Check sheet for the modelled part. Datum: model origin and axes. Units: mm. Face numbers are marked on the shaded views. A direction names the side the tool comes from. Round coordinates to 2 decimals unless told otherwise and drop trailing zeros. Write each loop counter-clockwise with the first axis right and the second up, starting at its lowest first coordinate (ties: lowest second). Pieces come first, ordered by that corner, then holes. Notation, with made-up numbers: M 12,17 L 22,17 A26 cw 22,37 Z; hole C 40,-19.5 d1. An arc over 180 degrees is marked long. One line per item, written item: value.
from build123d import *

# Parameters (mm, degrees)
SKETCH1_W           = 10.795
SKETCH1_H           = 10.795
BOSS_EXTRUDE1_DEPTH = 6.2992
SKETCH3_R           = 5.7404
BOSS_EXTRUDE2_DEPTH = 3
SKETCH4_R           = 2.8194
BOSS_EXTRUDE3_DEPTH = 19.939
SKETCH5_R           = 0.8255
CUT_EXTRUDE1_DEPTH  = 15
SKETCH7_R           = 3.2385
BOSS_EXTRUDE4_DEPTH = 10
SKETCH8_W           = 4.31
SKETCH8_H           = 1.016
BOSS_EXTRUDE5_DEPTH = 1


with BuildPart() as part:
    # Sketch1 → Boss-Extrude1 (new body)
    with BuildSketch(Plane(origin=(0, 0, 0), x_dir=(1, 0, 0), z_dir=(0, 1, 0))):
        Rectangle(SKETCH1_W, SKETCH1_H)
    extrude(amount=BOSS_EXTRUDE1_DEPTH)

    # Sketch3 → Boss-Extrude2 (add)
    with BuildSketch(Plane(origin=(0, 6.2992, 0), x_dir=(1, 0, 0), z_dir=(0, 1, 0))):
        Circle(SKETCH3_R)
    extrude(amount=-BOSS_EXTRUDE2_DEPTH)

    # Sketch4 → Boss-Extrude3 (add)
    with BuildSketch(Plane(origin=(0, 0, 0), x_dir=(1, 0, 0), z_dir=(0, 1, 0))):
        Circle(SKETCH4_R)
    extrude(amount=BOSS_EXTRUDE3_DEPTH)

    # Sketch5 → Cut-Extrude1 (cut)
    with BuildSketch(Plane(origin=(0, 19.939, 0), x_dir=(1, 0, 0), z_dir=(0, 1, 0))):
        Circle(SKETCH5_R)
    extrude(amount=-CUT_EXTRUDE1_DEPTH, mode=Mode.SUBTRACT)

    # Sketch7 → Boss-Extrude4 (add)
    with BuildSketch(Plane(origin=(0, 0, 0), x_dir=(1, 0, 0), z_dir=(0, 1, 0))):
        Circle(SKETCH7_R)
    extrude(amount=BOSS_EXTRUDE4_DEPTH)

    # Sketch8 → Boss-Extrude5 (add)
    with BuildSketch(Plane(origin=(0, 0, 0), x_dir=(1, 0, 0), z_dir=(0, 1, 0))):
        with Locations((-7.0525, 3.81)):
            Rectangle(SKETCH8_W, SKETCH8_H)
        with Locations((-7.0525, 1.27)):
            Rectangle(SKETCH8_W, SKETCH8_H)
        with Locations((-7.0525, -1.27)):
            Rectangle(SKETCH8_W, SKETCH8_H)
        with Locations((-7.0525, -3.81)):
            Rectangle(SKETCH8_W, SKETCH8_H)
        with Locations((7.0525, -3.81)):
            Rectangle(SKETCH8_W, SKETCH8_H)
        with Locations((7.0525, -1.27)):
            Rectangle(SKETCH8_W, SKETCH8_H)
        with Locations((7.0525, 1.27)):
            Rectangle(SKETCH8_W, SKETCH8_H)
        with Locations((7.0525, 3.81)):
            Rectangle(SKETCH8_W, SKETCH8_H)
    extrude(amount=BOSS_EXTRUDE5_DEPTH)


solid = part.part
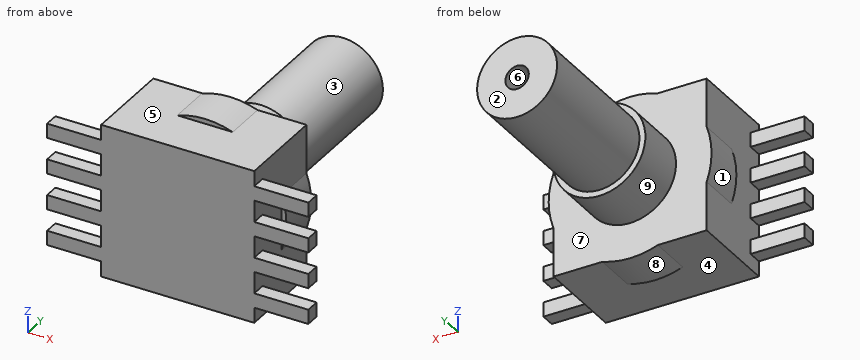
Q1. Scan lines: line 1 (X direction, y = 14.75, z = 0); line 2 (Y direction, x = -0.75, z = 4.5). Record each from-to range of solid material in increasing order. Write a range as [from, to].
Completed:
line 1: [-2.82, -0.83], [0.83, 2.82]
line 2: [0, 6.3]
Q2. Sectioned sample at C-C on y = 5.25. Enter the section's corners in (x, z).
Completed:
outline: M -5.4,-5.4 L -1.95,-5.4 A5.74 ccw 1.95,-5.4 L 5.4,-5.4 L 5.4,-1.95 A5.74 ccw 5.4,1.95 L 5.4,5.4 L 1.95,5.4 A5.74 ccw -1.95,5.4 L -5.4,5.4 L -5.4,1.95 A5.74 ccw -5.4,-1.95 Z
Q3. Draft check along Z on the marked faces 6, 7, 8 and 9. Enter one of: pulls with the +Z half, pulls with the -Z half, needs draft (parallel to the pull), parting line crosses it, or undercut.
Completed:
face 6: undercut
face 7: needs draft
face 8: pulls with the -Z half
face 9: parting line crosses it
Q4. Sectioned sample at D-D on x = 0. Enter the section's corners in (y, z), and give its area (3 significant figures).
Completed:
outline: M 0,-5.4 L 3.3,-5.4 L 3.3,-5.74 L 6.3,-5.74 L 6.3,-3.24 L 10,-3.24 L 10,-2.82 L 19.94,-2.82 L 19.94,-0.83 L 10,-0.83 L 10,0.83 L 19.94,0.83 L 19.94,2.82 L 10,2.82 L 10,3.24 L 6.3,3.24 L 6.3,5.74 L 3.3,5.74 L 3.3,5.4 L 0,5.4 Z
area: 134 mm^2
Q5. Sectioned sample at A-A on x = -6. Enter the section's corners in (y, z), and give its area (3 significant figures).
Completed:
outline: M 0,-4.32 L 1,-4.32 L 1,-3.3 L 0,-3.3 Z; M 0,-1.78 L 1,-1.78 L 1,-0.76 L 0,-0.76 Z; M 0,0.76 L 1,0.76 L 1,1.78 L 0,1.78 Z; M 0,3.3 L 1,3.3 L 1,4.32 L 0,4.32 Z
area: 4.06 mm^2
Q6. Depth check by flat-ended pin: P1, Ø0.5, axis at x = -7, y = 0.5, coming from the -Z side; P2, Ø6, axis at x = -1, y = 17.5, coming from the -Z side; P3, Ø1, axis at x = 2.5, y = 13, coming from the -Z side; P4, Ø1, axis at x = -7, y = 3.5, coming from the -Z side (3 decimals). Enter the tip coordinate at first touch or a pass-through.
Completed:
P1: z = -4.32
P2: z = -2.82
P3: z = -1.99
P4: through
Q7. Sectioned sample at B-B on z = 0. Enter the section's corners in (x, y), and give its area (3 significant figures).
Completed:
outline: M -5.74,3.3 L -5.4,3.3 L -5.4,0 L 5.4,0 L 5.4,3.3 L 5.74,3.3 L 5.74,6.3 L 3.24,6.3 L 3.24,10 L 2.82,10 L 2.82,19.94 L 0.83,19.94 L 0.83,10 L -0.83,10 L -0.83,19.94 L -2.82,19.94 L -2.82,10 L -3.24,10 L -3.24,6.3 L -5.74,6.3 Z
area: 134 mm^2
Q8. Access from +Z, -Z, +X, -X, +Y, -Y to the whole of each face (thin tool, end or side, straight path). Record for the marked faces 1, 2, 3, 4 and 5.
Completed:
face 1: -X, +Y
face 2: +Z, -Z, +X, -X, +Y
face 3: +Y
face 4: -Z, -Y
face 5: +Z, -Y
